Verification items for the finished model (mm, model axes). A direction names the side the tool comes from. Coordinates: 2 decimals unless noted, no trailing zeros. Order: outer loops, then holes, each group sorted by start corner. A loop starts at its lowest first (then second) coordinate and runs counter-clockwise, first axis right, second up.
Q1. Draft check along X on faces 1 (the cylindrical face through (-0.444, 1.999, -2.958)), 2 (the cylindrical face through (0.33, 0.74, -22.507)), 3 (the flat face through (0, 0, -18)), 4 (the cylindrical face through (12.698, 3.944, -39.317)). Enter one of: pulls with the +X half, pulls with the -X half, needs draft (parallel to the pull), parting line crosses it, or undercut.
Q2. Thickness scan on line 1 (Y direction, x = -10, z = -3.95); line 2 (Y direction, x = -1, z = -43); line 3 (Y direction, x = 8.5, z = -28.5). Record the ranges inside material, lowest first.
Q3. Depth check by flat-ended pin: P1, Ø1.5, axis at x = -10.5, y = 5.5, coming from the -Z side; P2, Ø2, axis at x = -11.91, z = -23.12, coming from the +Y side; P3, Ø1.5, axis at x = 1.5, y = 4.5, coming from the -Z side; P4, Ø13.5, axis at x = 0, z = -30, coming from the +Y side. Enter the tip coordinate at first touch or a pass-through.
Q4. Cross-section at A-A, the plane z = -2.5. Record the boundary of the cut face in (x, y).
Q5. Cross-section at B-B, the plane z = -43.75. Record the boundary of the cut face in (x, y), and give its area (3 significant figures).
Q6. Cross-section at C-C, the plane y = 4.5. Count the separate pieces of the cut face and the enclosed holes in it, and give its area (3 significant figures).
Q7. Set-up check for faces 5 (the cylindrical face through (12.05, 3.91, -2.96)), 6 (the flat face through (0, 8, -19)), 7 (the cylindrical face through (-0.67, 6.028, -42.133)): record each of +Z, -Z, +X, -X, +Y, -Y from which the full face is reachable in a straight line by a thin tool's end or side.
from build123d import *

# Parameters (mm, degrees)
SKETCH_1_R          = 9.75
EXTRUDE_1_DEPTH     = 8
SKETCH_2_R          = 2.05
CUT_EXTRUDE_1_DEPTH = 6
SKETCH_4_R          = 9.75
SKETCH_4_R_2        = 7.5
EXTRUDE_2_DEPTH     = 1.5
EXTRUDE_START       = -8
EXTRUDE_3_DEPTH     = 8
SKETCH_6_R          = 1.75
CUT_EXTRUDE_2_DEPTH = 4
FILLET_1_R          = 10
CHAMFER_1_SIZE      = 1


with BuildPart() as part:
    # Эскиз1 → Бобышка-Вытянуть1 (new body)
    with BuildSketch(Plane(origin=(0, 0, 0), x_dir=(1, 0, 0), z_dir=(0, 1, 0))):
        with BuildLine():
            Line((-15.75, 0), (15.75, 0))
            Line((15.75, 0), (15.75, 30))
            ThreePointArc((15.75, 30), (0, 45.75), (-15.75, 30))
            Line((-15.75, 30), (-15.75, 0))
        make_face()
        with Locations(Location((0, 30, 0), (0, 0, 270))):
            Circle(SKETCH_1_R, mode=Mode.SUBTRACT)
    extrude(amount=EXTRUDE_1_DEPTH)

    # Эскиз2 → Вырез-Вытянуть1 (cut)
    with BuildSketch(Plane.XY):
        with Locations((0, 4)):
            Circle(SKETCH_2_R)
        with Locations((-10, 4)):
            Circle(SKETCH_2_R)
        with Locations(Location((10, 4, 0), (0, 0, 180))):
            Circle(SKETCH_2_R)
    extrude(amount=-CUT_EXTRUDE_1_DEPTH, mode=Mode.SUBTRACT)

    # Эскиз4 → Бобышка-Вытянуть2 (add)
    with BuildSketch(Plane.XZ):
        with Locations(Location((0, -30, 0), (0, 0, 270))):
            Circle(SKETCH_4_R)
        with Locations(Location((0, -30, 0), (0, 0, 270))):
            Circle(SKETCH_4_R_2, mode=Mode.SUBTRACT)
    extrude(amount=-EXTRUDE_2_DEPTH)

    # Эскиз5 → Бобышка-Вытянуть3 (add)
    with BuildSketch(Plane(origin=(0, 8, 0), x_dir=(1, 0, 0), z_dir=(0, 1, 0)).offset(EXTRUDE_START)):
        with BuildLine():
            ThreePointArc((2.595683542, 45.534636364), (0, 46.9), (-2.595683542, 45.534636364))
            ThreePointArc((-2.595683542, 45.534636364), (0, 45.75), (2.595683542, 45.534636364))
        make_face()
    extrude(amount=EXTRUDE_3_DEPTH)

    # Эскиз6 → Вырез-Вытянуть2 (cut)
    with BuildSketch(Plane(origin=(0, 8, 0), x_dir=(1, 0, 0), z_dir=(0, 1, 0))):
        with Locations(Location((0, 43.75, 0), (0, 0, 270))):
            Circle(SKETCH_6_R)
        with Locations(Location((11.907849302, 23.125, 0), (0, 0, 270))):
            Circle(SKETCH_6_R)
        with Locations(Location((-11.907849302, 23.125, 0), (0, 0, 270))):
            Circle(SKETCH_6_R)
    extrude(amount=-CUT_EXTRUDE_2_DEPTH, mode=Mode.SUBTRACT)

    # Скругление1
    fillet_1_edges = [part.edges().sort_by_distance(p)[0] for p in [
        (2.595683542, 4, -45.534636364),
        (-2.595683542, 4, -45.534636364),
    ]]
    fillet(fillet_1_edges, radius=FILLET_1_R)

    # Фаска1
    chamfer_1_edges = [part.edges().sort_by_distance(p)[0] for p in [
        (0, 8, -39.75),
    ]]
    chamfer(chamfer_1_edges, length=CHAMFER_1_SIZE)


solid = part.part
Check values:
1. face 1: undercut
1. face 2: undercut
1. face 3: needs draft
1. face 4: pulls with the +X half
2. line 1: y = 0 to 1.95, 6.05 to 8
2. line 2: y = 0 to 4
2. line 3: y = 0 to 1.5
3. P1: stops at z = -42.37
3. P2: stops at y = 4
3. P3: stops at z = -46.81
3. P4: passes through
4. outline: (-15.75, 0) - (15.75, 0) - (15.75, 8) - (-15.75, 8) - close; hole circle Ø4.1 at (-10, 4); hole circle Ø4.1 at (0, 4); hole circle Ø4.1 at (10, 4)
5. outline: (-7.68, 0) - (7.68, 0) - (7.68, 8) - (1.75, 8) - (1.75, 4) - (-1.75, 4) - (-1.75, 8) - (-7.68, 8) - close
5. area: 109 mm2
6. separate pieces: 1
6. enclosed holes: 4
6. area: 940 mm2
7. face 5: +Z
7. face 6: +Z, -Z, +X, -X, +Y
7. face 7: +Y
